Verification items for the finished model (mm, model axes). A direction names the side the tool comes from. Round coordinates to 2 decimals unless told otherwise and drop trailing zeros. Order: outer loops, then holes, each group sorted by start corner. A loop starts at its lowest first (then second) coordinate and runs counter-clockwise, first axis right, second up. Notation, with made-up numbers: (-31.75, -32.5) -> (12.25, -32.5) arc R13 ccw to (12.25, -28.5) -> close; hole circle Ø2 at (27, -35.75). An arc over 180 degrees is marked (long way). Put each result on its own line as item: value.
```python
from build123d import *

# Parameters (mm, degrees)
SKETCH1_R           = 45.25
SKETCH1_R_2         = 38.25
BOSS_EXTRUDE1_DEPTH = 92.5
BOSS_EXTRUDE2_START = -6.35
SKETCH2_R           = 38.25
SKETCH2_R_2         = 36.25
BOSS_EXTRUDE2_DEPTH = 100
CUT_EXTRUDE3_START  = -44
SKETCH6_R           = 39.25
SKETCH6_R_2         = 38.25
CUT_EXTRUDE3_DEPTH  = 44
SKETCH7_R           = 17.5
CUT_EXTRUDE4_DEPTH  = 113.478331247
SKETCH10_R          = 2.25
CUT_EXTRUDE5_DEPTH  = 113.47833141


with BuildPart() as part:
    # Sketch1 → Boss-Extrude1 (new, symmetric)
    with BuildSketch(Plane(origin=(0, 0, 0), x_dir=(1, 0, 0), z_dir=(0, 1, 0))):
        with Locations(Location((0, 0, 0), (0, 0, 270))):
            Circle(SKETCH1_R)
        with Locations(Location((0, 0, 0), (0, 0, 270))):
            Circle(SKETCH1_R_2, mode=Mode.SUBTRACT)
    extrude(amount=BOSS_EXTRUDE1_DEPTH, both=True)

    # Sketch2 → Boss-Extrude2 (add)
    with BuildSketch(Plane.XZ.offset(92.5).offset(BOSS_EXTRUDE2_START)):
        with Locations(Location((0, 0, 0), (0, 0, 270))):
            Circle(SKETCH2_R)
        with Locations(Location((0, 0, 0), (0, 0, 270))):
            Circle(SKETCH2_R_2, mode=Mode.SUBTRACT)
    extrude(amount=-BOSS_EXTRUDE2_DEPTH)

    # Sketch6 → Cut-Extrude3 (cut)
    with BuildSketch(Plane(origin=(0, 92.5, 0), x_dir=(1, 0, 0), z_dir=(0, 1, 0)).offset(CUT_EXTRUDE3_START)):
        with Locations(Location((0, 0, 0), (0, 0, 270))):
            Circle(SKETCH6_R)
        with Locations(Location((0, 0, 0), (0, 0, 90))):
            Circle(SKETCH6_R_2, mode=Mode.SUBTRACT)
    extrude(amount=CUT_EXTRUDE3_DEPTH, mode=Mode.SUBTRACT)

    # Sketch7 → Cut-Extrude4 (cut, through all)
    with BuildSketch(Plane(origin=(0, 0, 0), x_dir=(0, 0, -1), z_dir=(1, 0, 0))):
        with Locations(Location((0, 44.35, 0), (0, 0, 13.717970606))):
            Circle(SKETCH7_R)
    extrude(amount=-CUT_EXTRUDE4_DEPTH, mode=Mode.SUBTRACT)

    # Sketch10 → Cut-Extrude5 (cut, through all)
    with BuildSketch(Plane(origin=(0, 0, 0), x_dir=(-0.5735764363510474, 0, -0.819152044288991), z_dir=(0.819152044288991, 0, -0.5735764363510474))):
        with Locations(Location((0, 40, 0), (0, 0, 180))):
            Circle(SKETCH10_R)
        with Locations(Location((0, -40, 0), (0, 0, 180))):
            Circle(SKETCH10_R)
    cut_extrude5 = extrude(amount=CUT_EXTRUDE5_DEPTH, mode=Mode.SUBTRACT)

    # Mirror1: Cut-Extrude5 across plane
    add(cut_extrude5.mirror(Plane.XY), mode=Mode.SUBTRACT)


solid = part.part
```
Item 1: Sectioned sample at C-C, the plane y = -15.5. Record the boundary of the cut face in (x, z).
Geometry check:
outline: circle Ø90.5 at (0, 0); hole circle Ø72.5 at (0, 0)
Item 2: Tool access check on faces 1 (the face through (-34, 13.85, -14)), 2 (the face through (-34, -86.15, -14)), 3 (the face through (33.13, -42.23, 23.56)). Record the directions out of +Z, -Z, +X, -X, +Y, -Y that give a thin tool (end or side, any length) a straight path to the whole face; none if there is none.
Geometry check:
face 1: +Y
face 2: -Y
face 3: none
Item 3: Release check for a two-part mould opening along Y. For faces 4 (the face through (-39.538, 26.854, -0.366)), 5 (the face through (-37.34, -89.37, -8.29)), 6 (the face through (32.5, 48.5, -20.5)) record: pulls with the +Y half, pulls with the -Y half, needs draft (parallel to the pull), parting line crosses it, or undercut.
Geometry check:
face 4: undercut
face 5: needs draft
face 6: pulls with the +Y half
Item 4: Depth check by flat-ended pin: pin 1 Ø5 at (x, y) = (31, 60) entering from -Z; pin 2 Ø10 at (y, z) = (70, -1.5) entering from +X; pin 3 Ø2 at (y, z) = (65, -18) entering from +X. Enter the tip coordinate at first touch or a pass-through.
Geometry check:
pin 1: z = -35.15
pin 2: x = 45.25
pin 3: x = 41.94
Item 5: Material ranges on line 1 along X through (y, z) = (-88, 0); line 2 along Y through (x, z) = (-41, 0); line 3 along Y through (x, z) = (-39, 0), recorded low to high.
Geometry check:
line 1: -45.25 to -38.25, 38.25 to 45.25
line 2: -92.5 to 26.85, 61.85 to 92.5
line 3: -92.5 to 26.85
Item 6: Sectioned sample at A-A, the plane x = 0. Record the boundary of the cut face in (y, z).
Geometry check:
outline: (-92.5, -45.25) -> (92.5, -45.25) -> (92.5, -39.25) -> (48.5, -39.25) -> (48.5, -38.25) -> (13.85, -38.25) -> (13.85, -36.25) -> (-86.15, -36.25) -> (-86.15, -38.25) -> (-92.5, -38.25) -> close; (-92.5, 38.25) -> (-86.15, 38.25) -> (-86.15, 36.25) -> (13.85, 36.25) -> (13.85, 38.25) -> (48.5, 38.25) -> (48.5, 39.25) -> (92.5, 39.25) -> (92.5, 45.25) -> (-92.5, 45.25) -> close
Item 7: Sectioned sample at B-B, the plane z = 0. Record the boundary of the cut face in (x, y).
Geometry check:
outline: (-45.25, -92.5) -> (-38.25, -92.5) -> (-38.25, -86.15) -> (-36.25, -86.15) -> (-36.25, 13.85) -> (-38.25, 13.85) -> (-38.25, 26.85) -> (-45.25, 26.85) -> close; (-45.25, 61.85) -> (-39.25, 61.85) -> (-39.25, 92.5) -> (-45.25, 92.5) -> close; (36.25, -86.15) -> (38.25, -86.15) -> (38.25, -92.5) -> (45.25, -92.5) -> (45.25, 92.5) -> (39.25, 92.5) -> (39.25, 48.5) -> (38.25, 48.5) -> (38.25, 13.85) -> (36.25, 13.85) -> close
Item 8: Sectioned sample at D-D, the plane x = 12. Record the boundary of the cut face in (y, z).
Geometry check:
outline: (-92.5, -43.63) -> (92.5, -43.63) -> (92.5, -37.37) -> (48.5, -37.37) -> (48.5, -36.32) -> (13.85, -36.32) -> (13.85, -34.21) -> (-86.15, -34.21) -> (-86.15, -36.32) -> (-92.5, -36.32) -> close; (-92.5, 36.32) -> (-86.15, 36.32) -> (-86.15, 34.21) -> (13.85, 34.21) -> (13.85, 36.32) -> (48.5, 36.32) -> (48.5, 37.37) -> (92.5, 37.37) -> (92.5, 43.63) -> (-92.5, 43.63) -> close
